Build history of the part. All positions in model axes, mm. Face numbers are marked on the shaded views. A direction names the side the tool comes from. Give positions to 0.01 mm unless a question says otherwise; leave off trailing zeros. Loops run counter-clockwise (first coordinate to the right, second up) from the corner with the lowest first, then second, coordinate; pieces in that order, holes last. Notation, with made-up numbers: (-14.75, 21.25) - (-5.75, 21.25) arc R20 ccw to (-5.75, 60.25) - close; hole circle Ø10 at (-38, 28.25). An arc over 180 degrees is marked (long way). Return JSON: item names as keys, results as strings. Group by question number.
1) Slice it at B-B (x = 17.78). List the corners of the cut face in (y, z).
2) Drill centre lines: probe 1 along Z at (x, y) = (17.78, -29); probe 2 along X at (y, z) = (-94.5, -55.5); probe 3 along Y at (x, z) = (46.5, -53). Where is each one in solid material? Low to high. Write a range as from..to.
3) Slice it at A-A (z = -12). List the corners of the cut face in (x, y) (3 decimals), and give its area (3 significant figures).
4) Drop flat-ended pins along their axis: pin 1 (23 mm diameter, centred on x = -67.98, y = -60.37, fed in from +Z); pin 2 (8 mm diameter, centred on y = -42.5, z = -34, fed in from +X) (3 decimals); pin 3 (12 mm diameter, centred on y = -89.5, z = 38, fed in from +X); pin 4 (8 mm diameter, centred on x = 14.5, z = -42, fed in from -Y). Give the stop position or say it passes through.
5) Mould opens along Z. For the marked faces 1, 2, 3 and 4 say: released by +Z, released by -Z, zero draft, split by the parting line, or undercut.
6) 3-axis set-ups, long thin cutter, end or side, ignore diameter. For the marked faces 5, 6 and 7: which of +Z, -Z, +X, -X, +Y, -Y reach the whole face in a straight line?
7) Slice it at D-D (x = -21). List the corners of the cut face in (y, z), and give its area (3 significant figures).
8) Slice it at C-C (y = -80.5). List the corners of the cut face in (x, z), and give its area (3 significant figures).
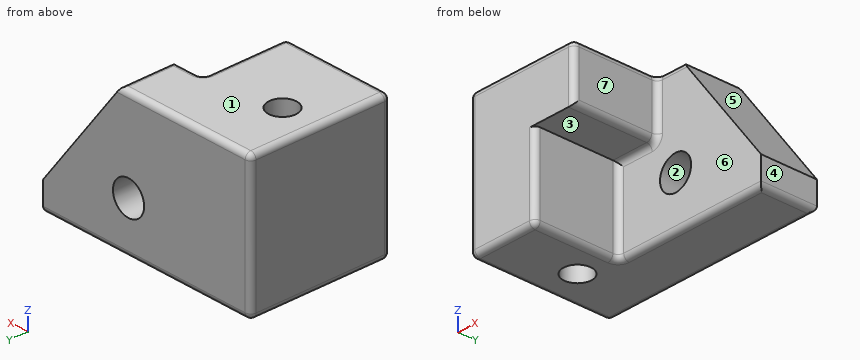
```python
from build123d import *

# Parameters (mm, degrees)
F0_W     = 203.2
F0_H     = 127
F1_DEPTH = 127
F3_DEPTH = 76.2
F4_SIZE2 = 101.6
F4_SIZE  = 76.2
F5_R     = 5.08
F6_R     = 15.24
F7_DEPTH = 50.8
F8_R     = 12.7
F9_DEPTH = 127


with BuildPart() as f1:
    # F0 (on Front) → F1 (new body)
    with BuildSketch(Plane.XZ):
        Rectangle(F0_W, F0_H)
    extrude(amount=F1_DEPTH)

    # F2 (on face) → F3 (cut)
    with BuildSketch(Plane.XZ.offset(127)):
        Polygon((101.6, 63.5), (0, 63.5), (0, 12.7), (-38.1, 12.7), (-38.1, -63.5), (101.6, -63.5), align=None)
    extrude(amount=-F3_DEPTH, mode=Mode.SUBTRACT)

    # F4
    f4_edges = [f1.edges().sort_by_distance(p)[0] for p in [
        (101.6, -25.4, 63.5),
    ]]
    f4_side = f1.faces().sort_by_distance((-21.771429, -52.614286, 63.5))[0]
    chamfer(f4_edges, length=F4_SIZE, length2=F4_SIZE2, reference=f4_side)

    # F5
    f5_edges = [f1.edges().sort_by_distance(p)[0] for p in [
        (0, -88.9, 63.5),
        (12.7, -50.8, 63.5),
        (25.4, -25.4, 63.5),
        (-38.1, 0, 63.5),
        (-101.6, -63.5, 63.5),
        (-50.8, -127, 63.5),
        (0, -127, 38.1),
        (0, -88.9, 12.7),
        (0, -50.8, 38.1),
        (-38.1, -50.8, -25.4),
        (-38.1, -127, -25.4),
        (-38.1, -88.9, -63.5),
        (-69.85, -127, -63.5),
        (-101.6, -127, 0),
        (31.75, -50.8, -63.5),
        (101.6, -25.4, -63.5),
        (-101.6, -63.5, -63.5),
        (-101.6, 0, 0),
        (0, 0, -63.5),
        (-19.05, -50.8, 12.7),
    ]]
    fillet(f5_edges, radius=F5_R)

    # F6 (on face) → F7 (cut, through all)
    with BuildSketch(Plane.XZ.offset(50.8)):
        with Locations((17.78, -17.78)):
            Circle(F6_R)
    extrude(amount=-F7_DEPTH, mode=Mode.SUBTRACT)

    # F8 (on face) → F9 (cut, through all)
    with BuildSketch(Plane.XY.offset(63.5)):
        with Locations((-67.9840967059, -60.368321836)):
            Circle(F8_R)
    extrude(amount=-F9_DEPTH, mode=Mode.SUBTRACT)


solid = f1.part
```
Results:
{
 "1": {"outline": "(-50.8, -58.42) arc R5.08 ccw to (-45.72, -63.5) - (-5.08, -63.5) arc R5.08 ccw to (0, -58.42) - (0, -33.02) - (-50.8, -33.02) - close; (-50.8, -2.54) - (0, -2.54) - (0, 58.42) arc R5.08 ccw to (-5.08, 63.5) - (-45.72, 63.5) arc R5.08 ccw to (-50.8, 58.42) - close"},
 "2": {"probe 1": "-63.5..-33.02, -2.54..63.5", "probe 2": "-101.6..-38.1", "probe 3": "-50.8..0"},
 "3": {"outline": "(-101.6, -121.92) arc R5.08 ccw to (-96.52, -127) - (-43.18, -127) arc R5.08 ccw to (-38.1, -121.92) - (-38.1, -55.88) arc R5.08 cw to (-33.02, -50.8) - (3.679, -50.8) - (3.679, 0) - (-96.52, 0) arc R5.08 ccw to (-101.6, -5.08) - close; (31.881, -50.8) - (82.025, -50.8) - (82.025, 0) - (31.881, 0) - close; hole circle Ø25.4 at (-67.984, -60.368)", "area": "12,200 mm2"},
 "4": {"pin 1": "through", "pin 2": "x = 101.525", "pin 3": "x = 0", "pin 4": "y = -50.8"},
 "5": {"face 1": "released by +Z", "face 2": "undercut", "face 3": "released by -Z", "face 4": "zero draft"},
 "6": {"face 5": "+Z, +X, +Y, -Y", "face 6": "-Z, +X, -Y", "face 7": "+Z, -Z, +X, -Y"},
 "7": {"outline": "(-127, 12.7) - (-55.88, 12.7) arc R5.08 cw to (-50.8, 7.62) - (-50.8, -58.42) arc R5.08 ccw to (-45.72, -63.5) - (-5.08, -63.5) arc R5.08 ccw to (0, -58.42) - (0, 58.42) arc R5.08 ccw to (-5.08, 63.5) - (-121.92, 63.5) arc R5.08 ccw to (-127, 58.42) - close", "area": "10,300 mm2"},
 "8": {"outline": "(-101.6, -58.42) arc R5.08 ccw to (-96.52, -63.5) - (-43.18, -63.5) arc R5.08 ccw to (-38.1, -58.42) - (-38.1, 12.7) - (-5.08, 12.7) arc R5.08 ccw to (0, 17.78) - (0, 58.42) arc R5.08 ccw to (-5.08, 63.5) - (-96.52, 63.5) arc R5.08 ccw to (-101.6, 58.42) - close", "area": "9,970 mm2"}
}
